Source: CAD feature listing. Evaluate the final solid. Frame: model axes, mm. Face numbers are marked on the shaded views. A direction names the side the tool comes from. Coordinates: 2 decimals unless noted, no trailing zeros. Order: outer loops, then holes, each group sorted by start corner. A loop starts at its lowest first (then second) coordinate and runs counter-clockwise, first axis right, second up.
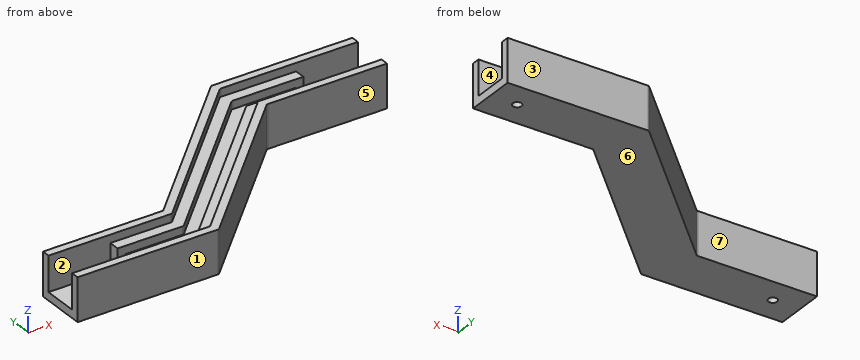
```python
from build123d import *

# Parameters (mm, degrees)
SKETCH_10_R     = 1.65
EXTRUDE_1_DEPTH = 3
EXTRUDE_START   = 3
EXTRUDE_2_DEPTH = 7
EXTRUDE_3_DEPTH = 13
CHAMFER_1_SIZE  = 7
EXTRUDE_5_DEPTH = 10
FILLET_1_R      = 1


with BuildPart() as part:
    # 草图10 → 凸台-拉伸1 (new body)
    with BuildSketch(Plane.XY):
        Polygon((-76.15, -18.05), (-31.485028843, -18.05), (23.614971157, 37.05), (76.15, 37.05), (76.15, 18.05), (31.485028843, 18.05), (-23.614971157, -37.05), (-76.15, -37.05), align=None)
        with Locations((-66.15, -27.55)):
            Circle(SKETCH_10_R, mode=Mode.SUBTRACT)
        with Locations((66.15, 27.55)):
            Circle(SKETCH_10_R, mode=Mode.SUBTRACT)
    extrude(amount=EXTRUDE_1_DEPTH)

    # 草图11 → 凸台-拉伸2 (add)
    with BuildSketch(Plane.XY.offset(EXTRUDE_START)):
        Polygon((-57.15, -18.05), (-57.15, -37.05), (-23.614971157, -37.05), (31.485028843, 18.05), (57.15, 18.05), (57.15, 37.05), (23.614971157, 37.05), (-31.485028843, -18.05), align=None)
    extrude(amount=EXTRUDE_2_DEPTH)

    # 草图12 → 凸台-拉伸3 (add)
    with BuildSketch(Plane.XY.offset(EXTRUDE_START)):
        Polygon((-76.15, -18.05), (-31.485028843, -18.05), (23.614971157, 37.05), (76.15, 37.05), (76.15, 34.05), (24.857611845, 34.05), (-30.242388155, -21.05), (-76.15, -21.05), align=None)
        Polygon((-76.15, -34.05), (-76.15, -37.05), (-23.614971157, -37.05), (31.485028843, 18.05), (76.15, 18.05), (76.15, 21.05), (30.242388155, 21.05), (-24.857611845, -34.05), align=None)
    extrude(amount=EXTRUDE_3_DEPTH)

    # 倒角1
    chamfer_1_edges = [part.edges().sort_by_distance(p)[0] for p in [
        (57.15, 27.55, 10),
        (-57.15, -27.55, 10),
    ]]
    chamfer(chamfer_1_edges, length=CHAMFER_1_SIZE - 0.0001)  # a hair under: the kernel refuses the full size

    # 草图15 → 凸台-拉伸5 (add)
    with BuildSketch(Plane.XY.offset(3)):
        Polygon((-53.15, -21.05), (-53.15, -25.05), (-28.585533906, -25.05), (26.514466094, 30.05), (53.15, 30.05), (53.15, 34.05), (24.857611845, 34.05), (-30.242388155, -21.05), align=None)
        Polygon((-53.15, -30.05), (-53.15, -34.05), (-24.857611845, -34.05), (30.242388155, 21.05), (53.15, 21.05), (53.15, 25.05), (28.585533906, 25.05), (-26.514466094, -30.05), align=None)
    extrude(amount=EXTRUDE_5_DEPTH)

    # 圆角1
    fillet_1_edges = [part.edges().sort_by_distance(p)[0] for p in [
        (-31.485028843, -18.05, 8),
        (23.614971157, 37.05, 8),
        (31.485028843, 18.05, 8),
        (-23.614971157, -37.05, 8),
        (-28.585533906, -25.05, 11.5),
        (26.514466094, 30.05, 11.5),
        (-26.514466094, -30.05, 11.5),
        (28.585533906, 25.05, 11.5),
        (24.857611845, 34.05, 14.5),
        (-30.242388155, -21.05, 14.5),
        (-24.857611845, -34.05, 14.5),
        (30.242388155, 21.05, 14.5),
    ]]
    fillet(fillet_1_edges, radius=FILLET_1_R)


solid = part.part
```
Q1. Pin query (flat end, axial travel): P1, Ø1.8, axis at x = -40.5, z = 10.5, coming from the +Y side; P2, Ø1, axis at y = -10, z = 12, coming from the +X side (3 decimals); P3, Ø3, axis at y = -32.5, z = 10.5, coming from the -X side; P4, Ø3, axis at x = -66.15, y = -27.55, coming from the +Z side. Return the tip coordinate at first contact, or that it passes through.
Solutions:
P1: stops at y = -18.05
P2: stops at x = 3.935
P3: stops at x = -53.15
P4: passes through
Q2. Pull-direction query (Y, two-part tool) for the marked faces 1, 2 and 3; classes: pulls with the +Y half, pulls with the -Y half, needs draft (parallel to the pull), parting line crosses it, or undercut.
Solutions:
face 1: pulls with the -Y half
face 2: undercut
face 3: pulls with the +Y half
Q3. Section query C-C on x = 39. Output: boundary loops of the cut face in (y, z).
Solutions:
outline: (18.05, 0) - (37.05, 0) - (37.05, 16) - (34.05, 16) - (34.05, 13) - (30.05, 13) - (30.05, 10) - (25.05, 10) - (25.05, 13) - (21.05, 13) - (21.05, 16) - (18.05, 16) - close
Q4. Material intervals for line 1 along Y through (x, z) = (66.15, 1.7); line 2 along Y through (x, z) = (-66.15, 1.7); line 3 along Z through (x, y) = (4, 0), sorted ascending.
Solutions:
line 1: y = 18.05 to 25.9, 29.2 to 37.05
line 2: y = -37.05 to -29.2, -25.9 to -18.05
line 3: z = 0 to 13
Q5. Section query B-B on x = 66.15. Output: boundary loops of the cut face in (y, z).
Solutions:
outline: (18.05, 0) - (25.9, 0) - (25.9, 3) - (21.05, 3) - (21.05, 16) - (18.05, 16) - close; (29.2, 0) - (37.05, 0) - (37.05, 16) - (34.05, 16) - (34.05, 3) - (29.2, 3) - close
Q6. Set-up query: the marked faces 4, 5, 6 and 7. Return all of +Z, -Z, +X, -X, +Y, -Y with unobstructed straight access to the full face (end or side cutting, diameter ignored); none if empty.
Solutions:
face 4: +Z, +X
face 5: +Z, -Z, +X, -Y
face 6: -Z, +X, -X, +Y, -Y
face 7: +Z, -Z, -X, +Y
